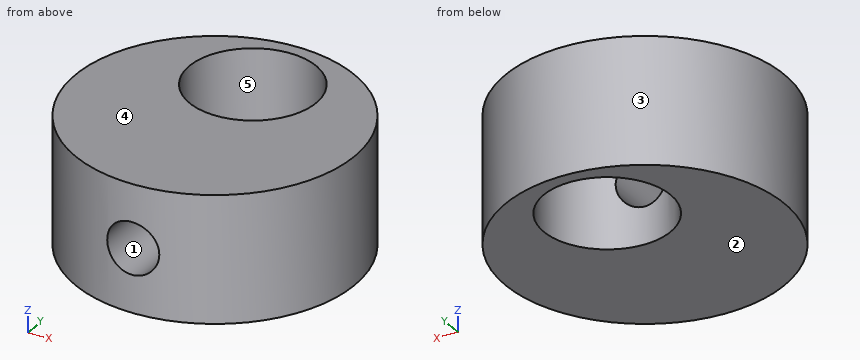
from build123d import *

# Parameters (mm, degrees)
SKETCH1_R               = 5.5
BOSS_EXTRUDE1_DEPTH     = 5
SKETCH4_R               = 2.5
CUT_EXTRUDE1_DEPTH      = 10.246621004
M2_5_TAPPED_HOLE2_D     = 2.05
M2_5_TAPPED_HOLE2_DEPTH = 8


with BuildPart() as part:
    # Sketch1 → Boss-Extrude1 (new body)
    with BuildSketch(Plane.XY):
        Circle(SKETCH1_R)
    extrude(amount=BOSS_EXTRUDE1_DEPTH)

    # Sketch4 → Cut-Extrude1 (cut, through all)
    with BuildSketch(Plane(origin=(0, 0, 0), x_dir=(-1, 0, 0), z_dir=(0, 0, -1))):
        with Locations((0, 2.5)):
            Circle(SKETCH4_R)
    extrude(amount=-CUT_EXTRUDE1_DEPTH, mode=Mode.SUBTRACT)

    # M2.5 Tapped Hole2
    with Locations(Plane(origin=(0, -5.5, 2.5), x_dir=(-1, 0, 0), z_dir=(0, -1, 0))):
        with Locations((0, 0)):
            Hole(M2_5_TAPPED_HOLE2_D / 2, depth=M2_5_TAPPED_HOLE2_DEPTH)


solid = part.part
Read the model definition and answer for the solid it produces. Units are mm, in the model's axes. Face numbers are marked on the shaded views. A direction names the side the tool comes from. Round coordinates to 2 decimals unless told otherwise and drop trailing zeros. Write each loop counter-clockwise with the first axis right and the second up, starting at its lowest first coordinate (ties: lowest second). Pieces come first, ordered by that corner, then holes.
1. Which of the six approach directions +Z, -Z, +X, -X, +Y, -Y give full straight-line access (tool end or side, diameter ignored) to the marked faces 1 and 2?
2. The part is cut by section B-B, the plane y = 2.5. Determine the outline of the cut face in (x, z).
3. The part is cut by section A-A, the plane x = 0. Determine the outline of the cut face in (y, z) (3 decimals).
4. The part is cut by section D-D, the plane y = -3.5. Determine the outline of the cut face in (x, z) (3 decimals).
5. The part is cut by section C-C, the plane z = 3.95. Determine the outline of the cut face in (x, y).
6. Given pin 1 Ø1.5 at (y, z) = (-0.5, 2) entering from +X; pin 2 Ø1.5 at (x, z) = (-4, 4.5) entering from -Y; pin 3 Ø1.2 at (x, z) = (0, 2.5) entering from -Y, each flat-ended and moving along its own axis, determine where each tip first touches the part or whether it passes through.
7. Straight lines are drawn through the part: L1, parallel to Z at x = 0, y = -1.65 (3 decimals); L2, parallel to Y at x = 0, z = 3.8; L3, parallel to X at y = 2, z = 3.2. For each, find the intervals that lie inside material, in ascending order.
8. Determine the mould class of the marked faces 3, 4 and 5 for opening direction Y: pulls with the +Y half, pulls with the -Y half, needs draft (parallel to the pull), parting line crosses it, or undercut.
Values:
1. face 1: -Y
1. face 2: -Z, +X, -X, +Y, -Y
2. outline: (-4.9, 0) - (-2.5, 0) - (-2.5, 5) - (-4.9, 5) - close; (2.5, 0) - (4.9, 0) - (4.9, 5) - (2.5, 5) - close
3. outline: (-5.5, 0) - (0, 0) - (0, 1.475) - (-5.5, 1.475) - close; (-5.5, 3.525) - (0, 3.525) - (0, 5) - (-5.5, 5) - close; (5, 0) - (5.5, 0) - (5.5, 5) - (5, 5) - close
4. outline: (-4.243, 0) - (4.243, 0) - (4.243, 5) - (-4.243, 5) - close; hole circle Ø2.05 at (0, 2.5)
5. outline: circle Ø11 at (0, 0); hole circle Ø5 at (0, 2.5)
6. pin 1: stops at x = 5.5
6. pin 2: stops at y = -4.44
6. pin 3: stops at y = 4.93
7. L1: z = 0 to 1.475, 3.525 to 5
7. L2: y = -5.5 to 0, 5 to 5.5
7. L3: x = -5.12 to -2.45, 2.45 to 5.12
8. face 3: parting line crosses it
8. face 4: needs draft
8. face 5: undercut
